Study the drawing (mm; zero at the part's minimum x, y, z) and answer. A direction names the side the tool comes from. Give positions to 0.01 mm unless a question says otherwise; leave off trailing zeros. Order: outer loops, then holes, each group sorted by start corner. A loop starts at its lowest first (then second) coordinate and runs counter-clockwise, first axis right, second up.
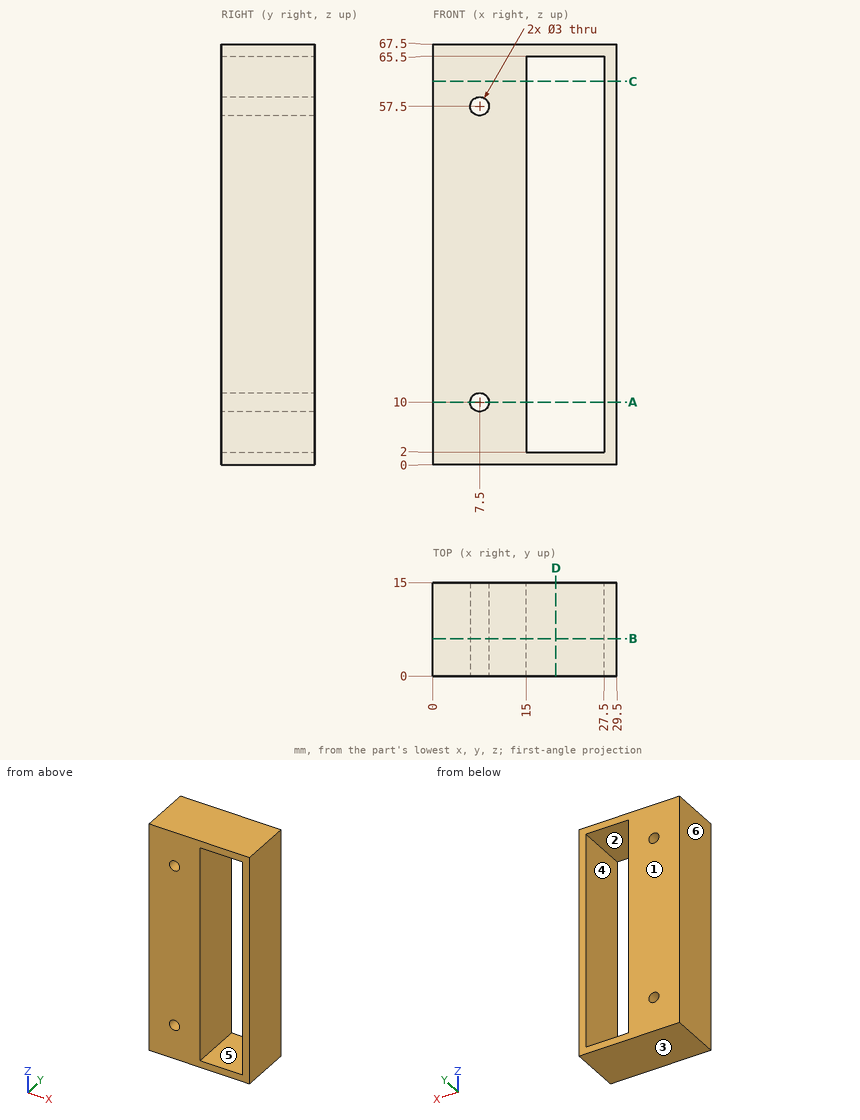
1) Find section D-D (x = 19.75). Write down the section's boundary in (y, z), then the cut area to 3 significant figures.
Geometry says:
outline: (0, 0) - (15, 0) - (15, 2) - (0, 2) - close; (0, 65.5) - (15, 65.5) - (15, 67.5) - (0, 67.5) - close
area: 60.0 mm2
2) Straight lines are drawn through the part: probe 1 along X at (y, z) = (7.75, 57.5); probe 2 along Z at (x, y) = (20.25, 6); probe 3 along X at (y, z) = (9, 41.5). For each, find the intervals that lie inside material, in ascending order.
Geometry says:
probe 1: x = 0 to 6, 9 to 15, 27.5 to 29.5
probe 2: z = 0 to 2, 65.5 to 67.5
probe 3: x = 0 to 15, 27.5 to 29.5
3) For a pull along X with two mould halves and no side action, classify the marked faces 3, 4, 5 and 6 as +X half, -X half, draft (parallel to the pull), parting line (faces both ways), or undercut.
Geometry says:
face 3: draft
face 4: undercut
face 5: undercut
face 6: -X half
4) Find section C-C (z = 61.5). Write down the section's boundary in (x, y).
Geometry says:
outline: (0, 0) - (15, 0) - (15, 15) - (0, 15) - close; (27.5, 0) - (29.5, 0) - (29.5, 15) - (27.5, 15) - close
5) Find section A-A (z = 10). Write down the section's boundary in (x, y), then the cut area to 3 significant figures.
Geometry says:
outline: (0, 0) - (6, 0) - (6, 15) - (0, 15) - close; (9, 0) - (15, 0) - (15, 15) - (9, 15) - close; (27.5, 0) - (29.5, 0) - (29.5, 15) - (27.5, 15) - close
area: 210 mm2
6) A tool of negligible diameter and unlimited length cuts with its end or side. For the marked faces 1 and 2, from which of +Z, -Z, +X, -X, +Y, -Y can it reach the whole face along a straight path? Write none if from no direction.
Geometry says:
face 1: +Z, -Z, +X, -X, +Y
face 2: +Y, -Y
7) Find section B-B (y = 6). Write down the section's boundary in (x, z).
Geometry says:
outline: (0, 0) - (29.5, 0) - (29.5, 67.5) - (0, 67.5) - close; hole circle Ø3 at (7.5, 10); hole circle Ø3 at (7.5, 57.5); hole (15, 2) - (27.5, 2) - (27.5, 65.5) - (15, 65.5) - close
8) Given P1, Ø1.8, axis at x = 7.5, z = 57.5, coming from the -Y side, flat-ended and moving along its own axis, determine where the tip first touches the part or whether it passes through.
Geometry says:
P1: passes through
